Geometry: final body of the model. Coordinates: model frame, mm. A direction names the side the tool comes from. Give positions to 0.01 mm unless a question says otherwise; leave off trailing zeros. Loops run counter-clockwise (first coordinate to the right, second up) from the corner with the lowest first, then second, coordinate; pieces in that order, holes last.
1. Material intervals for line 1 along X through (y, z) = (12.5, 48.5); line 2 along Z through (x, y) = (40.5, 25); line 3 along X through (y, z) = (19.5, 24.5), sorted ascending.
2. Section B-B, the plane y = 25. Output: boundary loops of the cut face in (x, z).
3. Section C-C, the plane x = 14. Output: boundary loops of the cut face in (y, z).
4. Access query for faces 1 (the face through (0, 25, 25)), 2 (the face through (50, 25, 9)), 3 (the face through (25, 40, 25)). Directions: +Z, -Z, +X, -X, +Y, -Y. A direction counts if a zero-diameter tool reaches every point of the face in a straight line with its end or side. Return the directions, or none.
5. First-contact query: P1, Ø15, axis at x = 27, z = 27, coming from the +Y side; P2, Ø1.5, axis at x = 1.5, z = 36.5, coming from the -Y side; P3, Ø4.5, axis at y = 23.5, z = 21.5, coming from the +X side; P4, Ø6, axis at x = 1.5, z = 38, coming from the +Y side. Flat tips, straight axial feed; report the tip coordinate or a pass-through.
6. Section A-A, the plane z = 19. Output: boundary loops of the cut face in (x, y).
7. Section D-D, the plane y = 3.5. Output: boundary loops of the cut face in (x, z).
8. Draft query along X for faces 4 (the face through (-10, 25, 25)), 5 (the face through (55.07, 2.85, 3.01)), 6 (the face through (25, 25, 10)). Return one class per face: +X half, -X half, draft (parallel to the pull), parting line (faces both ways), or undercut.
Autodesk Inventor part; units mm, degrees
ref_plane "YZ Plane" through (0, 0, 0) normal (1, 0, 0) x (0, 1, 0)
ref_plane "XZ Plane" through (0, 0, 0) normal (0, 1, 0) x (-1, 0, 0)
ref_plane "XY Plane" through (0, 0, 0) normal (0, 0, 1) x (1, 0, 0)
sketch "Sketch1" plane through (0, 0, 0) normal (1, 0, 0) x (0, 1, 0)
  line L0 (0, 0) -> (50, 0)
  line L1 (50, 0) -> (50, 50)
  line L2 (50, 50) -> (0, 50)
  line L3 (0, 50) -> (0, 0)
  circle A0 centre (25, 25) radius 7.5
  dimension "d0" = 50
  dimension "d1" = 50
  dimension "d2" = 15
extrude "Extrusion1" add sketch "Sketch1" along normal blind 60
extrude "Extrusion7" add sketch "Sketch1" against normal blind 10 contours L3 L2 L1 L0 | A0
sketch "Sketch6" plane through (60, 0, 50) normal (0, 0, 1) x (1, 0, 0)
  line L0 (0, 50) -> (-70, 50)
  line L1 (-70, 0) -> (0, 0)
  line L2 (-60, 50) -> (-10, 50)
  line L3 (-10, 50) -> (-10, 0)
  line L4 (-10, 0) -> (-60, 0)
  line L5 (-60, 0) -> (-60, 50)
  line L6 (-60, 50) -> (-10, 50)
  line L7 (-10, 50) -> (-10, 40)
  line L8 (-10, 40) -> (-60, 40)
  line L9 (-60, 40) -> (-60, 50)
  line L10 (-10, 0) -> (-60, 0)
  line L11 (-60, 0) -> (-60, 10)
  line L12 (-60, 10) -> (-10, 10)
  line L13 (-10, 10) -> (-10, 0)
  line L14 (-60, 50) -> (-10, 50)
  line L15 (-10, 50) -> (-10, 0)
  line L16 (-10, 0) -> (-60, 0)
  line L17 (-60, 0) -> (-60, 50)
  point P0 (-10, 10)
  dimension "d33" = 50
  dimension "d34" = 10
  dimension "d35" = 10
extrude "Extrusion8" cut sketch "Sketch6" against normal blind 100 contours L3 L8 L5 L0 | L3 L1 L5 L12
extrude "Extrusion9" cut sketch "Sketch6" against normal blind 10 contours L3 L12 L5 L8
sketch "Sketch7" plane through (60, 0, 0) normal (0, 0, -1) x (-1, 0, 0)
  line L0 (60, 10) -> (60, 40)
  line L1 (10, 0) -> (10, 10)
  line L2 (60, 40) -> (10, 40)
  line L3 (10, 40) -> (10, 10)
  line L4 (10, 10) -> (60, 10)
  line L5 (60, 10) -> (60, 40)
  point P0 (60, 0)
extrude "Extrusion10" cut sketch "Sketch7" against normal blind 10
fillet "Fillet4" radius 10 8 edges at (55, 50, 50) (-5, 50, 50) (-5, 50, 0) (55, 0, 50) (55, 50, 0) (-5, 0, 50) (55, 0, 0) (-5, 0, 0)
sketch "Sketch8" plane through (60, 0, 0) normal (1, 0, 0) x (0, 0, -1)
  point P0 (0, 0)
properties part number "Contenedor"
Answers below:
1. line 1: x = -10 to 0, 50 to 60
1. line 2: z = 10 to 17.5, 32.5 to 40
1. line 3: x = -10 to 0
2. outline: (-10, 0) - (0, 0) - (0, 10) - (50, 10) - (50, 0) - (60, 0) - (60, 17.5) - (0, 17.5) - (0, 32.5) - (60, 32.5) - (60, 50) - (50, 50) - (50, 40) - (0, 40) - (0, 50) - (-10, 50) - close
3. outline: (10, 10) - (40, 10) - (40, 40) - (10, 40) - close; hole circle Ø15 at (25, 25)
4. face 1: +X
4. face 2: none
4. face 3: +Z, -Z, +Y
5. P1: stops at y = 40
5. P2: stops at y = 10
5. P3: stops at x = 0
5. P4: stops at y = 50
6. outline: (-10, 0) - (0, 0) - (0, 10) - (50, 10) - (50, 0) - (60, 0) - (60, 20.5) - (0, 20.5) - (0, 29.5) - (60, 29.5) - (60, 50) - (50, 50) - (50, 40) - (0, 40) - (0, 50) - (-10, 50) - close
7. outline: (-10, 2.4) - (0, 2.4) - (0, 47.6) - (-10, 47.6) - close; (50, 2.4) - (60, 2.4) - (60, 47.6) - (50, 47.6) - close
8. face 4: -X half
8. face 5: draft
8. face 6: undercut
